Autodesk Inventor part; units mm, degrees
ref_plane "YZ Plane" through (0, 0, 0) normal (1, 0, 0) x (0, 1, 0)
ref_plane "XZ Plane" through (0, 0, 0) normal (0, 1, 0) x (-1, 0, 0)
ref_plane "XY Plane" through (0, 0, 0) normal (0, 0, 1) x (1, 0, 0)
sketch "Sketch1" plane through (0, 0, 0) normal (0, 0, 1) x (1, 0, 0)
  arc A0 (165, 0) -> (-165, 0) centre (0, 0) ccw
  line L0 (-165, 0) -> (-165, -100)
  line L1 (165, 0) -> (165, -100)
  arc A1 (-165, 0) -> (165, 0) centre (0, 0) ccw construction
  arc A2 (115, 0) -> (-115, 0) centre (0, 0) ccw
  line L2 (-115, 0) -> (-115, -100)
  line L3 (-115, -100) -> (-165, -100)
  line L4 (165, -100) -> (115, -100)
  line L5 (115, -100) -> (115, 0)
  arc A3 (-115, 0) -> (115, 0) centre (0, 0) ccw construction
  dimension "d0" = 330
  dimension "d1" = 100
  dimension "d2" = 100
  dimension "d4" = 230
extrude "Extrusion1" add sketch "Sketch1" along normal blind 10
sketch "Sketch2" plane through (0, 0, 10) normal (0, 0, 1) x (1, 0, 0)
  arc A0 (160, 0) -> (-160, 0) centre (0, 0) ccw
  arc A1 (155, 0) -> (-155, 0) centre (0, 0) ccw
  line L0 (-160, 0) -> (-160, -100)
  line L1 (-165, -100) -> (-115, -100)
  line L2 (-155, 0) -> (-155, -100)
  line L3 (155, 0) -> (155, -100)
  line L4 (115, -100) -> (165, -100)
  line L5 (160, 0) -> (160, -100)
  point P0 (160, -100)
  dimension "d7" = 320
  dimension "d8" = 310
extrude "Extrusion2" cut sketch "Sketch2" against normal blind 3
properties part number "Tapa Frontar y Posterior" material "Acrylic"
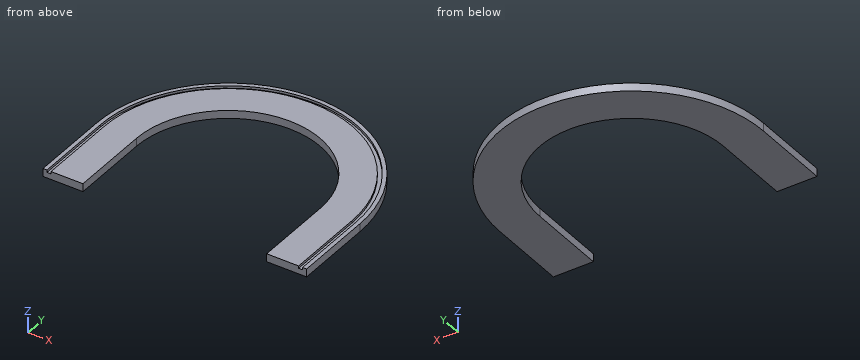
Model file for the job. Use its own axes, mm. Give positions to 0.01 mm unless a question says otherwise; leave off trailing zeros. Write each loop counter-clockwise with the first axis right and the second up, starting at its lowest first coordinate (ties: lowest second). Pieces come first, ordered by that corner, then holes. Notation, with made-up numbers: M 42.25,69.25 L 74.25,69.25 A18 cw 74.25,84.25 Z; hole C 37.5,56.25 d6. An arc over 180 degrees is marked long. One line per item, written item: value. Start each with the question number.
Q1. Saw through at D-D, the plane y = 64. Write the cut outline in (x, z).
Q2. Saw through at C-C, the plane x = -26. Write the cut outline in (y, z), plus the area to 3 significant figures.
Q3. Saw through at B-B, the plane z = 2.25. Write the cut outline in (x, y), plus the area to 3 significant figures.
Q4. Probe probe 1 along X at (y, z) = (-32.5, 8.75); probe 2 along X at (y, z) = (-16, 3.25); probe 3 along X at (y, z) = (88.5, 6.25). List the from-to ranges inside material, lowest first. Write a range as [from, to].
Q5. Drop flat-ended pins along their axis: pin 1 Ø2 at (x, z) = (-88.5, 5.5) entering from -Y; pin 2 Ø5 at (x, z) = (55, 4.5) entering from +Y; pin 3 Ø1 at (x, z) = (-80.5, 2.5) entering from +Y. Give the stop position or say it passes through.
Q6. Saw through at A-A, the plane y = -63. Write the cut outline in (x, z).
Output values:
1. outline: M -152.08,0 L -95.55,0 L -95.55,10 L -141.17,10 L -141.17,7 L -146.64,7 L -146.64,10 L -152.08,10 Z; M 95.55,0 L 152.08,0 L 152.08,10 L 146.64,10 L 146.64,7 L 141.17,7 L 141.17,10 L 95.55,10 Z
2. outline: M 112.02,0 L 162.94,0 L 162.94,10 L 157.87,10 L 157.87,7 L 152.8,7 L 152.8,10 L 112.02,10 Z
2. area: 494 mm²
3. outline: M -165,-100 L -115,-100 L -115,0 A115 cw 115,0 L 115,-100 L 165,-100 L 165,0 A165 ccw -165,0 Z
3. area: 32,000 mm²
4. probe 1: x = [-165, -160], [-155, -115], [115, 155], [160, 165]
4. probe 2: x = [-165, -115], [115, 165]
4. probe 3: x = [-139.26, -73.44], [73.44, 139.26]
5. pin 1: stops at y = 72.21
5. pin 2: stops at y = 156.42
5. pin 3: stops at y = 144.31
6. outline: M -165,0 L -115,0 L -115,10 L -155,10 L -155,7 L -160,7 L -160,10 L -165,10 Z; M 115,0 L 165,0 L 165,10 L 160,10 L 160,7 L 155,7 L 155,10 L 115,10 Z
